```python
from build123d import *

# Parameters (mm, degrees)
F1_DEPTH = 75
F3_DEPTH = 25


with BuildPart() as f1:
    # F0 (on Top) → F1 (new body)
    with BuildSketch(Plane.XY):
        Polygon((0, 50), (0, 0), (40.5, 0), (40.5, 15), (70, 15), (70, 10), (100, 10), (100, -20), (120, -20), (120, 50), align=None)
    extrude(amount=F1_DEPTH)

    # F2 (on face) → F3 (cut)
    with BuildSketch(Plane.XY.offset(75)):
        Polygon((23, 50), (23, 0), (40.5, 0), (40.5, 15), (70, 15), (70, 10), (90, 10), (90, 50), align=None)
    extrude(amount=-F3_DEPTH, mode=Mode.SUBTRACT)


solid = f1.part
```
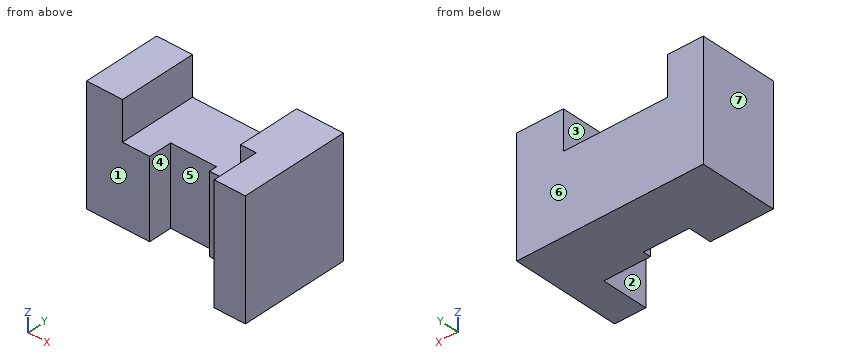
Here's how the part is built. I have some questions about the finished solid (model axes, mm). Face numbers are marked on the shaded views. A direction names the side the tool comes from. Give positions to 0.01 mm unless a question says otherwise; leave off trailing zeros. Write each loop counter-clockwise with the first axis right and the second up, starting at its lowest first coordinate (ties: lowest second). Pieces come first, ordered by that corner, then holes.
(1) If I drill on L1, parallel to X at y = 12, z = 5; L2, parallel to X at y = 0.5, z = 5; L3, parallel to X at y = -1, z = 10, over which ranges is the centre line in solid material (lowest first)?
Output values:
L1: x = 0 to 40.5, 70 to 120
L2: x = 0 to 40.5, 100 to 120
L3: x = 100 to 120
(2) On a 3-axis mill with a long thin cutter (end or side, diameter ignored), from which of +Z, -Z, +X, -X, +Y, -Y can I reach the whole of each face in a straight line? I mean the marked faces 1, 2 and 3. Say none if no direction works.
Output values:
face 1: +Z, -Z, -X, -Y
face 2: +Z, -Z, -Y
face 3: +Z, +Y, -Y
(3) Imagine slicing it at D-D, the plane z = 34. Write out the boundary of the cut face in (x, y).
Output values:
outline: (0, 0) - (40.5, 0) - (40.5, 15) - (70, 15) - (70, 10) - (100, 10) - (100, -20) - (120, -20) - (120, 50) - (0, 50) - close
(4) Thinking about a two-plate mould opening in X: for the marked faces 4, 5, 6 and 7, which applies, pulls with the +X half, pulls with the -X half, needs draft (parallel to the pull), parting line crosses it, or undercut?
Output values:
face 4: undercut
face 5: undercut
face 6: needs draft
face 7: pulls with the -X half
(5) Imagine slicing it at C-C, the plane y = 40.5. Write out the boundary of the cut face in (x, z).
Output values:
outline: (0, 0) - (120, 0) - (120, 75) - (90, 75) - (90, 50) - (23, 50) - (23, 75) - (0, 75) - close
(6) Will these pins go through, and if not, where does the flat tip stop? pin 1 (7.5 mm diameter, centred on y = 29.5, z = 59.5, fed in from -X); pin 2 (12 mm diameter, centred on x = 18, z = 28, fed in from -Y); pin 3 (25 mm diameter, centred on x = 59.5, y = 21, fed in from +Z); pin 4 (9 mm diameter, centred on x = 57, z = 34, fed in from -Y).
Output values:
pin 1: stops at x = 0
pin 2: stops at y = 0
pin 3: stops at z = 50
pin 4: stops at y = 15
(7) Imagine slicing it at A-A, the plane z = 69. Write out the boundary of the cut face in (x, y), and give its area (3 significant figures).
Output values:
outline: (0, 0) - (23, 0) - (23, 50) - (0, 50) - close; (90, 10) - (100, 10) - (100, -20) - (120, -20) - (120, 50) - (90, 50) - close
area: 2,950 mm2
(8) Imagine slicing it at B-B, the plane y = 1.5. Write out the boundary of the cut face in (x, z).
Output values:
outline: (0, 0) - (40.5, 0) - (40.5, 50) - (23, 50) - (23, 75) - (0, 75) - close; (100, 0) - (120, 0) - (120, 75) - (100, 75) - close
